```python
from build123d import *

# Parameters (mm, degrees)
F0_R     = 8.365692
F0_R_2   = 7.949673
F1_DEPTH = 76.2


with BuildPart() as f1:
    # F0 (on Front) → F1 (new body)
    with BuildSketch(Plane.XZ):
        Polygon((-4.221705, 28.852343), (-4.221705, 0), (71.978295, 0), (71.978295, 28.852343), (11.756951, 28.852343), align=None)
        with Locations((33.878295, 14.426172)):
            Circle(F0_R, mode=Mode.SUBTRACT)
        with Locations((55.086598, 13.778679)):
            Circle(F0_R_2, mode=Mode.SUBTRACT)
        with BuildLine():
            Line((-26.343049, 28.852343), (-4.221705, 28.852343))
            Line((-4.221705, 28.852343), (11.756951, 28.852343))
            Line((11.756951, 28.852343), (11.756951, 53.244089))
            Line((11.756951, 53.244089), (-19.993049, 53.244089))
            ThreePointArc((-19.993049, 53.244089), (-24.483177, 51.384217), (-26.343049, 46.894089))
            Line((-26.343049, 46.894089), (-26.343049, 28.852343))
        make_face()
    extrude(amount=F1_DEPTH)


solid = f1.part
```
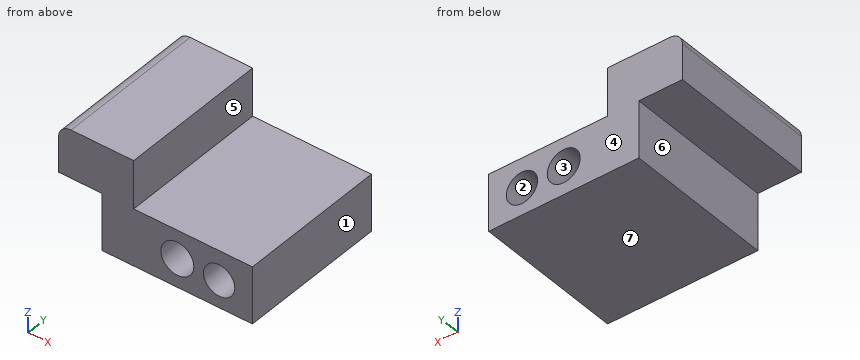
The listing builds one solid part. Answer for the finished solid, in the listing's coordinates (mm). Face numbers are marked on the shaded views. A direction names the side the tool comes from. Give positions to 0.01 mm unless a question says otherwise; leave off trailing zeros. Order: outer loops, then holes, each group sorted by start corner. A loop starts at its lowest first (then second) coordinate and runs counter-clockwise, first axis right, second up. Notation, with made-up numbers: M -16,-19.75 L -8,-19.75 A24 cw -8,8.25 Z; hole C 78,36 d5. An arc over 180 degrees is marked long. Put each result on its own line as item: value. Start each with the question number.
Item 1: The part is cut by section C-C, the plane y = -13.5. Determine the outline of the cut face in (x, z), and give its area (3 significant figures).
Item 2: Which of the six approach directions +Z, -Z, +X, -X, +Y, -Y give full straight-line access (tool end or side, diameter ignored) to the marked faces 5, 6 and 7?
Item 3: The part is cut by section D-D, the plane z = 41. Determine the outline of the cut face in (x, y).
Item 4: Find the intervals of material crossed by line 1 along X through (y, z) = (-58, 29.5); line 2 along Z through (x, y) = (56.5, -8.5); line 3 along Z through (x, y) = (-18, -64), in increasing order.
Item 5: The part is cut by section A-A, the plane z = 8. Determine the outline of the cut face in (x, y), and give its area (3 significant figures).
Item 6: Flat-ended cylindrical pins translate along their axes: P1, Ø12, axis at x = 47, y = -14, coming from the +Z side; P2, Ø5, axis at y = -46, z = 32.5, coming from the +X side; P3, Ø14.5, axis at y = -21, z = 17.5, coming from the -X side; P4, Ø9.5, axis at x = 55.09, z = 13.78, coming from the -Y side. Find the tip coordinate at first contact, or state that the pin passes through.
Item 7: The part is cut by section B-B, the plane x = 36. Determine the outline of the cut face in (y, z), and give its area (3 significant figures).
Item 8: For a pull along X with two mould halves and no side action, classify the marked faces 1, 2, 3 and 4 as +X half, -X half, draft (parallel to the pull), parting line (faces both ways), or undercut.
Answer key:
1. outline: M -26.34,28.85 L -4.22,28.85 L -4.22,0 L 71.98,0 L 71.98,28.85 L 11.76,28.85 L 11.76,53.24 L -19.99,53.24 A6.35 ccw -26.34,46.89 Z; hole C 33.88,14.43 d16.73; hole C 55.09,13.78 d15.9
1. area: 2,700 mm²
2. face 5: +Z, +X, +Y, -Y
2. face 6: -Z, -X, +Y, -Y
2. face 7: -Z, +X, -X, +Y, -Y
3. outline: M -26.34,-76.2 L 11.76,-76.2 L 11.76,0 L -26.34,0 Z
4. line 1: x = -26.34 to 11.76
4. line 2: z = 0 to 5.96, 21.6 to 28.85
4. line 3: z = 28.85 to 53.24
5. outline: M -4.22,-76.2 L 28.52,-76.2 L 28.52,0 L -4.22,0 Z; M 39.23,-76.2 L 49.63,-76.2 L 49.63,0 L 39.23,0 Z; M 60.55,-76.2 L 71.98,-76.2 L 71.98,0 L 60.55,0 Z
5. area: 4,160 mm²
6. P1: stops at z = 28.85
6. P2: stops at x = 11.76
6. P3: stops at x = -4.22
6. P4: passes through
7. outline: M -76.2,0 L 0,0 L 0,6.33 L -76.2,6.33 Z; M -76.2,22.52 L 0,22.52 L 0,28.85 L -76.2,28.85 Z
7. area: 965 mm²
8. face 1: +X half
8. face 2: undercut
8. face 3: undercut
8. face 4: draft
